```python
from build123d import *

# Parameters (mm, degrees)
BOSS_EXTRUDE1_DEPTH = 30.5
SKETCH4_W           = 23.4
SKETCH4_H           = 10
CUT_EXTRUDE2_DEPTH  = 25
CUT_EXTRUDE4_DEPTH  = 11.5
SKETCH7_W           = 31
SKETCH7_H           = 1.7
BOSS_EXTRUDE3_DEPTH = 9.100050305
BOSS_EXTRUDE4_DEPTH = 9.100050305
LPATTERN1_COUNT     = 9
LPATTERN1_PITCH     = 3.4
SKETCH11_W          = 12
SKETCH11_H          = 4.5
BOSS_EXTRUDE5_DEPTH = 2
FILLET1_R           = 2
FILLET2_R           = 2
FILLET5_R           = 3
SKETCH12_W          = 2.5
SKETCH12_H          = 3.5
CUT_EXTRUDE5_DEPTH  = 12


with BuildPart() as part:
    # Sketch1 → Boss-Extrude1 (new body)
    with BuildSketch(Plane.XY):
        Polygon((0, 0), (0, -30), (12, -30), (12, -20), (5, 0), align=None)
    extrude(amount=-BOSS_EXTRUDE1_DEPTH)

    # Sketch4 → Cut-Extrude2 (cut)
    with BuildSketch(Plane.ZY):
        with Locations((-14.8, -25.899949695)):
            Rectangle(SKETCH4_W, SKETCH4_H)
    extrude(amount=-CUT_EXTRUDE2_DEPTH, mode=Mode.SUBTRACT)

    # Sketch6 → Cut-Extrude4 (cut, symmetric)
    with BuildSketch(Plane.XY.offset(-15.25)):
        Polygon((5, 0), (5, -14), (9.9, -14), align=None)
    extrude(amount=CUT_EXTRUDE4_DEPTH, both=True, mode=Mode.SUBTRACT)

    # Sketch7 → Boss-Extrude3 (add)
    with BuildSketch(Plane(origin=(0, -30, 0), x_dir=(1, 0, 0), z_dir=(0, 1, 0))):
        with Locations((-4.2231607, 26.1)):
            Rectangle(SKETCH7_W, SKETCH7_H)
    extrude(amount=BOSS_EXTRUDE3_DEPTH)

    # Sketch10 → Boss-Extrude4 (add)
    with BuildSketch(Plane(origin=(0, -20.899949695, 0), x_dir=(1, 0, 0), z_dir=(0, 1, 0))):
        Polygon((11.2768393, 25.25), (10.057972835, 22.860002615), (9.869194152, 22.860002615), (8.630940097, 25.25), align=None)
    boss_extrude4 = extrude(amount=-BOSS_EXTRUDE4_DEPTH)

    # LPattern1: Boss-Extrude4 ×9
    with Locations(*[(-i * LPATTERN1_PITCH, 0, 0) for i in range(1, LPATTERN1_COUNT)]):
        add(boss_extrude4)

    # Sketch11 → Boss-Extrude5 (add)
    with BuildSketch(Plane(origin=(0, 0, -30.5), x_dir=(-1, 0, 0), z_dir=(0, 0, -1))):
        with Locations((-6, -27.75)):
            Rectangle(SKETCH11_W, SKETCH11_H)
    boss_extrude5 = extrude(amount=BOSS_EXTRUDE5_DEPTH)

    # Fillet1
    fillet1_edges = [part.edges().sort_by_distance(p)[0] for p in [
        (6, -25.5, -32.5),
    ]]
    fillet(fillet1_edges, radius=FILLET1_R - 0.0001)  # a hair under: the kernel refuses the full size

    # Mirror1: Boss-Extrude5 across plane
    add(boss_extrude5.mirror(Plane.XY.offset(-15.25)))

    # Fillet2
    fillet2_edges = [part.edges().sort_by_distance(p)[0] for p in [
        (6, -25.5, 2),
    ]]
    fillet(fillet2_edges, radius=FILLET2_R - 0.0001)  # a hair under: the kernel refuses the full size

    # Fillet5
    fillet5_edges = [part.edges().sort_by_distance(p)[0] for p in [
        (5, -14, -15.25),
    ]]
    fillet(fillet5_edges, radius=FILLET5_R)

    # Sketch12 → Cut-Extrude5 (cut)
    with BuildSketch(Plane.ZY):
        with Locations((-29.713851252, -28.814354386)):
            Rectangle(SKETCH12_W, SKETCH12_H)
        with Locations((-0.786148748, -28.814354386)):
            Rectangle(SKETCH12_W, SKETCH12_H)
    extrude(amount=-CUT_EXTRUDE5_DEPTH, mode=Mode.SUBTRACT)


solid = part.part
```
Input: part model. Units: mm. Frame: model coordinates. A direction names the side the tool comes from. Give positions to 0.01 mm unless a question says otherwise; leave off trailing zeros. Order: outer loops, then holes, each group sorted by start corner. A loop starts at its lowest first (then second) coordinate and runs counter-clockwise, first axis right, second up. Notation, with made-up numbers: (75, 78.5) - (110, 78.5) arc R10 ccw to (110, 84.5) - close; hole circle Ø4 at (83.25, 57.25). An arc over 180 degrees is marked (long way). Use a Markdown table: item, result.
(1) Section query A-A (z = -16). Output: boundary loops of the cut face in (x, y).
Computed values:
| item | result |
|---|---|
| outline | (0, -20.9) - (12, -20.9) - (12, -20) - (9.9, -14) - (8, -14) arc R3 cw to (5, -11) - (5, 0) - (0, 0) - close |
(2) Section query B-B (y = -3). Output: boundary loops of the cut face in (x, z).
Computed values:
| item | result |
|---|---|
| outline | (0, -30.5) - (6.05, -30.5) - (6.05, -26.75) - (5, -26.75) - (5, -3.75) - (6.05, -3.75) - (6.05, 0) - (0, 0) - close |
(3) Pin query (flat end, axial travel): pin 1 (2.5 mm diameter, centred on x = -5.5, y = -27.5, fed in from -Z); pin 2 (1.2 mm diameter, centred on x = -14, z = -24.5, fed in from +Y); pin 3 (9 mm diameter, centred on y = -13.5, z = -20.5, fed in from -X). Return the tip coordinate at first contact, or that it passes through.
Computed values:
| item | result |
|---|---|
| pin 1 | stops at z = -26.95 |
| pin 2 | stops at y = -20.9 |
| pin 3 | stops at x = 0 |
(4) Section query D-D (z = -29). Output: boundary loops of the cut face in (x, y), then the cut area to 3 significant figures.
Computed values:
| item | result |
|---|---|
| outline | (0, -27.06) - (12, -27.06) - (12, -20) - (5, 0) - (0, 0) - close |
| area | 255 mm2 |
(5) Line query: line 1 (Z direction, x = 3, y = -27.25); line 2 (Z direction, x = 4, y = -7.25); line 3 (X direction, y = -27, z = -31). Output: solid intervals per line, ascending. Write a range as from..to.
Computed values:
| item | result |
|---|---|
| line 1 | z = -32.48..-30.96, -28.46..-22.99, -3.1..-2.04, 0.46..1.98 |
| line 2 | z = -30.5..0 |
| line 3 | x = 0..12 |
(6) Draft query along Z for faces 4 (the cylindrical face through (5.92, -26.07, -31.9)), 5 (the flat face through (-16.524, -25.386, -24.072)), 6 (the flat face through (10.676, -25.386, -24.072)). Return one class per face: released by +Z, released by -Z, zero draft, split by the parting line, or undercut.
Computed values:
| item | result |
|---|---|
| face 4 | released by -Z |
| face 5 | released by +Z |
| face 6 | undercut |
(7) Access query for faces 1 (the flat face through (6, -29, -28.464)), 2 (the flat face through (6, -10, -26.75)), 3 (the flat face through (-6.324, -25.386, -24.072)). Directions: +Z, -Z, +X, -X, +Y, -Y. A direction counts if a zero-diameter tool reaches every point of the face in a straight line with its end or side. Return the directions, or none.
Computed values:
| item | result |
|---|---|
| face 1 | +X, -X, -Y |
| face 2 | +X, +Y |
| face 3 | +Z, +Y, -Y |
